Part model, mm, in its own coordinate system. Round coordinates to 2 decimals unless told otherwise and drop trailing zeros. Loops run counter-clockwise (first coordinate to the right, second up) from the corner with the lowest first, then second, coordinate; pieces in that order, holes last. Notation, with made-up numbers: M 5.5,65 L 51.5,65 A25 ccw 51.5,79 Z; hole C 64,45 d2. An arc over 180 degrees is marked long. Put each result on its own line as item: value. Start each with the question number.
1) Slice it at A-A on x = 18. Give the cut face in (y, z), then the cut area to 3 significant figures.
2) Slice it at C-C on x = 38. Give the cut face in (y, z), then the cut area to 3 significant figures.
3) Drop flat-ended pins along their axis: pin 1 Ø16.5 at (x, z) = (37, 63) entering from -Y; pin 2 Ø1 at (x, z) = (33, 35) entering from -Y. Give the stop position or say it passes through.
4) Slice it at D-D on z = 18.5. Give the cut face in (x, y).
5) Probe line 1 along X through (y, z) = (-7, 50.5); line 2 along Z through (x, y) = (32.5, -7.75); line 3 along Y through (x, z) = (30.5, 40.5). List the from-to ranges inside material, lowest first.
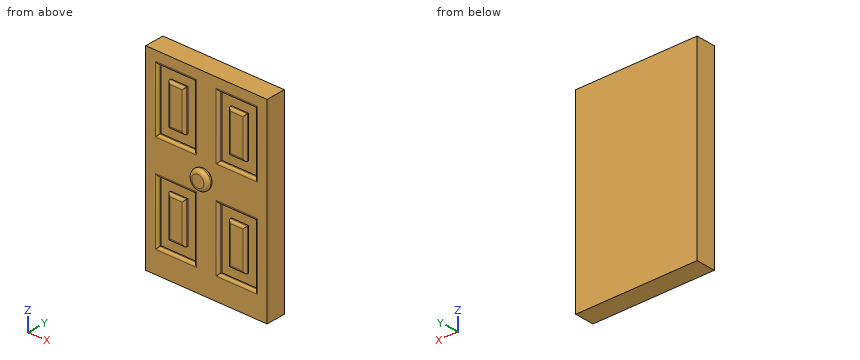
```python
from build123d import *

# Parameters (mm, degrees)
F0_W     = 50
F0_H     = 80
F1_DEPTH = 8
F2_W     = 15
F2_H     = 25
F2_W_2   = 7
F2_H_2   = 17
F3_DEPTH = 1.5
F4_R     = 1
F5_R     = 2
F6_DEPTH = 1
F7_R     = 4
F7_R_2   = 2
F8_DEPTH = 3
F9_R     = 1.49999


# Not quite as in the source:
# - a fillet or chamfer is up to 0.001 mm smaller than in the source, because OpenCascade refuses the exact size


with BuildPart() as f1:
    # F0 (on Front) → F1 (new body)
    with BuildSketch(Plane.XZ):
        with Locations((25, 40)):
            Rectangle(F0_W, F0_H)
    extrude(amount=F1_DEPTH)

    # F2 (on face) → F3 (cut)
    with BuildSketch(Plane.XZ.offset(8)):
        with Locations((12.5, 62.5)):
            Rectangle(F2_W, F2_H)
        with Locations((12.5, 62.5)):
            Rectangle(F2_W_2, F2_H_2, mode=Mode.SUBTRACT)
        with Locations((37.5, 62.5)):
            Rectangle(F2_W, F2_H)
        with Locations((37.5, 62.5)):
            Rectangle(F2_W_2, F2_H_2, mode=Mode.SUBTRACT)
        with Locations((12.5, 22.5)):
            Rectangle(F2_W, F2_H)
        with Locations((12.5, 22.5)):
            Rectangle(F2_W_2, F2_H_2, mode=Mode.SUBTRACT)
        with Locations((37.5, 22.5)):
            Rectangle(F2_W, F2_H)
        with Locations((37.5, 22.5)):
            Rectangle(F2_W_2, F2_H_2, mode=Mode.SUBTRACT)
    extrude(amount=-F3_DEPTH, mode=Mode.SUBTRACT)

    # F4
    f4_edges = [f1.edges().sort_by_distance(p)[0] for p in [
        (16, -8, 62.5),
        (12.5, -8, 71),
        (9, -8, 62.5),
        (12.5, -8, 54),
        (5, -8, 62.5),
        (12.5, -8, 75),
        (20, -8, 62.5),
        (12.5, -8, 50),
        (37.5, -8, 75),
        (45, -8, 62.5),
        (37.5, -8, 71),
        (30, -8, 62.5),
        (34, -8, 62.5),
        (41, -8, 62.5),
        (37.5, -8, 54),
        (37.5, -8, 50),
        (37.5, -8, 35),
        (37.5, -8, 31),
        (34, -8, 22.5),
        (37.5, -8, 14),
        (41, -8, 22.5),
        (45, -8, 22.5),
        (37.5, -8, 10),
        (30, -8, 22.5),
        (20, -8, 22.5),
        (16, -8, 22.5),
        (9, -8, 22.5),
        (5, -8, 22.5),
        (12.5, -8, 35),
        (12.5, -8, 31),
        (12.5, -8, 14),
        (12.5, -8, 10),
    ]]
    fillet(f4_edges, radius=F4_R)

    # F5 (on face) → F6 (join)
    with BuildSketch(Plane.XZ.offset(8)):
        with Locations((25, 43)):
            Circle(F5_R)
    extrude(amount=F6_DEPTH)

    # F7 (on face) → F8 (join)
    with BuildSketch(Plane.XZ.offset(9)):
        with Locations((25, 43)):
            Circle(F7_R)
        with Locations((25, 43)):
            Circle(F7_R_2, mode=Mode.SUBTRACT)
        with Locations((25, 43)):
            Circle(F7_R_2)
    extrude(amount=F8_DEPTH)

    # F9 (radius 1.5 in the source; OpenCascade refuses exactly that, so slightly less here)
    f9_edges = [f1.edges().sort_by_distance(p)[0] for p in [
        (21, -12, 43),
        (21, -9, 43),
    ]]
    fillet(f9_edges, radius=F9_R)


solid = f1.part
```
Recorded:
1. outline: M -8,0 L 0,0 L 0,80 L -8,80 L -8,76 A1 ccw -7,75 L -6.5,75 L -6.5,50 L -7,50 A1 ccw -8,49 L -8,36 A1 ccw -7,35 L -6.5,35 L -6.5,10 L -7,10 A1 ccw -8,9 Z
1. area: 564 mm2
2. outline: M -8,0 L 0,0 L 0,80 L -8,80 L -8,76 A1 ccw -7,75 L -6.5,75 L -6.5,71 L -7,71 A1 ccw -8,70 L -8,55 A1 ccw -7,54 L -6.5,54 L -6.5,50 L -7,50 A1 ccw -8,49 L -8,36 A1 ccw -7,35 L -6.5,35 L -6.5,31 L -7,31 A1 ccw -8,30 L -8,15 A1 ccw -7,14 L -6.5,14 L -6.5,10 L -7,10 A1 ccw -8,9 Z
2. area: 614 mm2
3. pin 1: stops at y = -8
3. pin 2: stops at y = -7.87
4. outline: M 0,-8 L 4,-8 A1 ccw 5,-7 L 5,-6.5 L 9,-6.5 L 9,-7 A1 ccw 10,-8 L 15,-8 A1 ccw 16,-7 L 16,-6.5 L 20,-6.5 L 20,-7 A1 ccw 21,-8 L 29,-8 A1 ccw 30,-7 L 30,-6.5 L 34,-6.5 L 34,-7 A1 ccw 35,-8 L 40,-8 A1 ccw 41,-7 L 41,-6.5 L 45,-6.5 L 45,-7 A1 ccw 46,-8 L 50,-8 L 50,0 L 0,0 Z
5. line 1: x = 0 to 5, 20 to 30, 45 to 50
5. line 2: z = 0 to 9.66, 35.34 to 49.66, 75.34 to 80
5. line 3: y = -8 to 0
